Verification items for the finished model (mm, model axes). A direction names the side the tool comes from. Coordinates: 2 decimals unless noted, no trailing zeros. Order: outer loops, then holes, each group sorted by start corner. A loop starts at its lowest first (then second) coordinate and runs counter-clockwise, first axis right, second up.
Q1. Cross-section at A-A, the plane z = 0. Record the boundary of the cut face in (x, y).
Q2. Set-up check for faces 1 (the flat face through (3, -0.529, -5)), 2 (the flat face through (0, 0.794, 0)): record each of +Z, -Z, +X, -X, +Y, -Y from which the full face is reachable in a straight line by a thin tool's end or side.
Q3. Cross-section at B-B, the plane y = 0.45. Record the boundary of the cut face in (x, z), and give its area (3 significant figures).
Q4. Draft check along Z on faces 3 (the flat face through (0, -0.794, 0)), 4 (the conical face through (-3.124, 0.319, -4.074)). Enter one of: pulls with the +Z half, pulls with the -Z half, needs draft (parallel to the pull), parting line crosses it, or undercut.
Q5. Depth check by flat-ended pin: P1, Ø2, axis at x = -4.5, z = -4.5, coming from the +Y side. Enter the tip coordinate at first touch or a pass-through.
Q6. Thickness scan on line 1 (Y direction, x = -5.25, z = -2); line 2 (X direction, y = -0.05, z = 4.25); line 3 (X direction, y = -0.1, z = -1). Record the ranges inside material, lowest first.
from build123d import *

# Parameters (mm, degrees)
FILLET1_R = 0.298588597
FILLET2_R = 0.059717719


with BuildPart() as part:
    # Sketch2 → Revolve1 (revolve)
    with BuildSketch(Plane(origin=(0, 0, 0), x_dir=(0, 0, -1), z_dir=(1, 0, 0))):
        with BuildLine():
            Line((-6.35, -0.79375), (-6.35, -0.529166667))
            Line((-6.35, -0.529166667), (-5.155645611, -0.529166667))
            Line((-5.155645611, -0.529166667), (-5.124404304, 0.663890696))
            ThreePointArc((-5.124404304, 0.663890696), (-5.084150358, 0.755918864), (-4.9911, 0.79375))
            Line((-4.9911, 0.79375), (0, 0.79375))
            Line((0, 0.79375), (0, -0.79375))
            Line((0, -0.79375), (-6.35, -0.79375))
        make_face()
    revolve(axis=Axis((0, -0.79375, 0), (0, 1, 0)))

    # Fillet1
    fillet1_edges = [part.edges().sort_by_distance(p)[0] for p in [
        (0, -0.529166667, -5.155645611),
    ]]
    fillet(fillet1_edges, radius=FILLET1_R)

    # Fillet2
    fillet2_edges = [part.edges().sort_by_distance(p)[0] for p in [
        (0, -0.529166667, -6.35),
    ]]
    fillet(fillet2_edges, radius=FILLET2_R)


solid = part.part
Check values:
1. outline: (-6.35, -0.79) - (6.35, -0.79) - (6.35, -0.59) arc R0.06 ccw to (6.29, -0.53) - (5.45, -0.53) arc R0.3 cw to (5.15, -0.24) - (5.12, 0.66) arc R0.13 ccw to (4.99, 0.79) - (-4.99, 0.79) arc R0.13 ccw to (-5.12, 0.66) - (-5.15, -0.24) arc R0.3 cw to (-5.45, -0.53) - (-6.29, -0.53) arc R0.06 ccw to (-6.35, -0.59) - close
2. face 1: +Y
2. face 2: +Z, -Z, +X, -X, +Y
3. outline: circle Ø10.26 at (0, 0)
3. area: 82.7 mm2
4. face 3: needs draft
4. face 4: parting line crosses it
5. P1: stops at y = -0.52
6. line 1: y = -0.79 to -0.53
6. line 2: x = -2.9 to 2.9
6. line 3: x = -5.05 to 5.05
